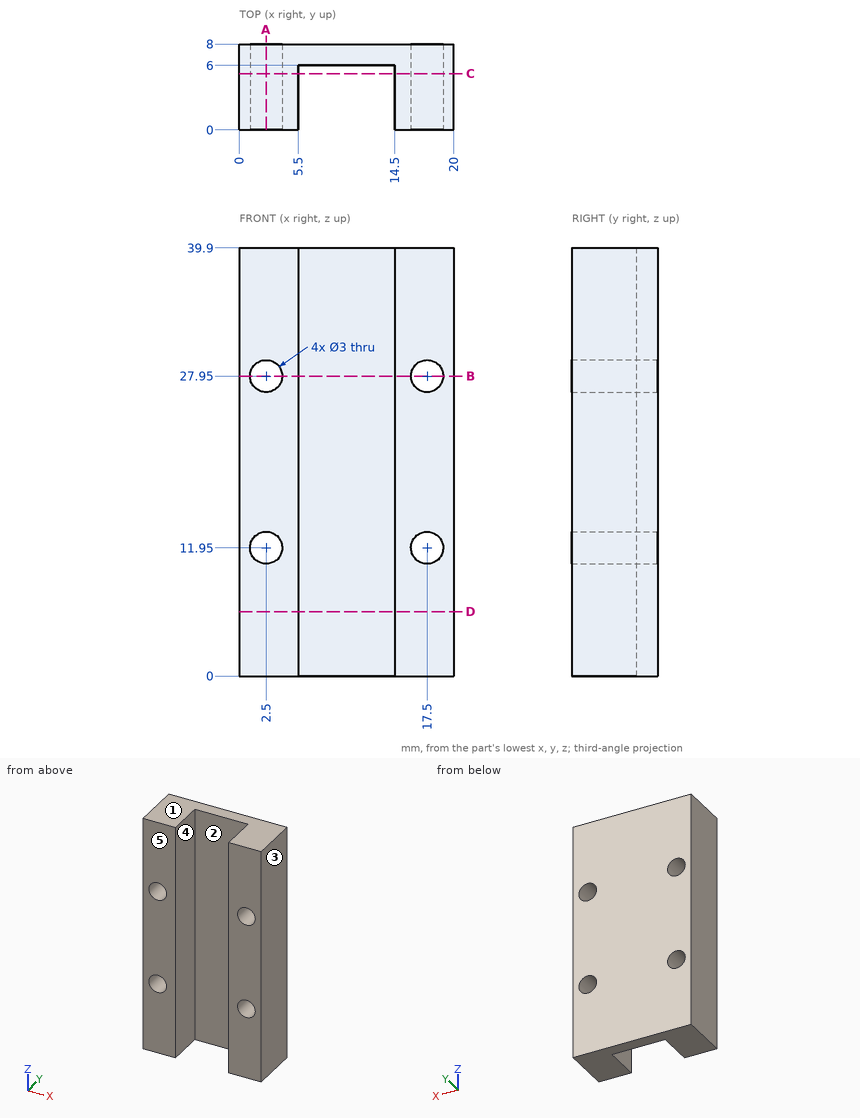
Here's the drawing with two shaded views (mm, measured from the low corner). I have some questions. A direction names the side the tool comes from. Coordinates: 2 decimals unless noted, no trailing zeros. Write each loop counter-clockwise with the first axis right and the second up, starting at its lowest first coordinate (ties: lowest second). Pieces come first, ordered by that corner, then holes. Notation, with made-up numbers: (16.5, 26) -> (72.5, 26) arc R28 cw to (72.5, 52) -> close; hole circle Ø6 at (-19, 0). An arc over 180 degrees is marked (long way). Write item = value, one per line. Start each with the question number.
(1) Which directions (+Z, -Z, +X, -X, +Y, -Y) give clear straight access to the entire face, cutting with the end or side of a thin tool? Please do the marked faces 4 and 5.
(2) Will this pin go through, and if not, where does the flat tip stop? pin 1 (4.5 mm diameter, centred on x = 10.5, z = 22.5, fed in from -Y).
(3) I need wall thicknesses on line 1 (X direction, y = 5.5, z = 27.95); line 2 (X direction, y = 4.25, z = 14.5); line 3 (Z direction, x = 3.5, y = 3.25). Which ranges of each line are inside material? Lowest first, please. Write a range as [from, to].
(4) I want a section at B-B (z = 27.95). Please give me the cut outline in (x, y).
(5) I want a section at C-C (y = 5.25). Please give me the cut outline in (x, z).
(6) I want a section at A-A (x = 2.5). Please give me the cut outline in (y, z), plus the area to 3 significant figures.
(7) I want a section at D-D (z = 6). Please give me the cut outline in (x, y).
(8) We'd pull the mould along X, two halves only. Please class the marked faces 1, 2 and 3: released by +X, released by -X, zero draft, split by the parting line, or undercut.
Result set:
q1.face_4 = +Z, -Z, -Y
q1.face_5 = +Z, -Z, +X, -X, -Y
q2.pin_1 = 6
q3.line_1 = [0, 1], [4, 5.5], [14.5, 16], [19, 20]
q3.line_2 = [0, 5.5], [14.5, 20]
q3.line_3 = [0, 10.83], [13.07, 26.83], [29.07, 39.9]
q4.outline = (0, 0) -> (1, 0) -> (1, 8) -> (0, 8) -> close; (4, 0) -> (5.5, 0) -> (5.5, 6) -> (14.5, 6) -> (14.5, 0) -> (16, 0) -> (16, 8) -> (4, 8) -> close; (19, 0) -> (20, 0) -> (20, 8) -> (19, 8) -> close
q5.outline = (0, 0) -> (5.5, 0) -> (5.5, 39.9) -> (0, 39.9) -> close; (14.5, 0) -> (20, 0) -> (20, 39.9) -> (14.5, 39.9) -> close; hole circle Ø3 at (2.5, 11.95); hole circle Ø3 at (2.5, 27.95); hole circle Ø3 at (17.5, 11.95); hole circle Ø3 at (17.5, 27.95)
q6.outline = (0, 0) -> (8, 0) -> (8, 10.45) -> (0, 10.45) -> close; (0, 13.45) -> (8, 13.45) -> (8, 26.45) -> (0, 26.45) -> close; (0, 29.45) -> (8, 29.45) -> (8, 39.9) -> (0, 39.9) -> close
q6.area = 271 mm2
q7.outline = (0, 0) -> (5.5, 0) -> (5.5, 6) -> (14.5, 6) -> (14.5, 0) -> (20, 0) -> (20, 8) -> (0, 8) -> close
q8.face_1 = zero draft
q8.face_2 = undercut
q8.face_3 = released by +X
